from build123d import *

# Parameters (mm, degrees)
F0_W     = 139.677039
F0_H     = 166.199392
F1_DEPTH = 13
F3_DEPTH = 8


# Not quite as in the source:
# - ends of sketch curves that miss each other by under 0.0002 mm in the source are joined


with BuildPart() as f1:
    # F0 (on Top) → F1 (new body)
    with BuildSketch(Plane.XY):
        with Locations((5e-07, 0)):
            Rectangle(F0_W, F0_H)
    extrude(amount=F1_DEPTH)

    # F2 (on face) → F3 (cut)
    with BuildSketch(Plane.XY.offset(13)):
        with BuildLine():
            Line((-52.224, 63.413361), (-52.224, -19.296639))
            ThreePointArc((-52.224, -19.296639), (-23.4870244983, -65.9411012245), (31.0980686358, -61.2520475086))
            Line((31.0980686358, -61.2520475086), (46.412829, -75.243303))
            Line((46.412829, -75.243303), (60.220039, -60.767602))
            Line((60.220039, -60.767602), (44.587774, -46.486281))
            ThreePointArc((44.587774, -46.486281), (50.2787135157, -33.4174443314), (52.224, -19.296639))
            Line((52.224, -19.296639), (52.224, 63.413361))
            Line((52.224, 63.413361), (35, 63.413361))
            Line((35, 63.413361), (35, -19.296639))
            ThreePointArc((35, -19.296639), (34.1157796878, -27.1141562719), (31.5077956402, -34.536678826))
            Line((31.5077956402, -34.536678826), (17.818477, -22.030395))
            Line((17.818477, -22.030395), (4.000974, -36.496692))
            Line((4.000974, -36.496692), (18.018091, -49.302445))
            ThreePointArc((18.018091, -49.302445), (-17.2390082984, -49.756720958), (-35, -19.296639))
            Line((-35, -19.296639), (-35, 63.413361))
            Line((-35, 63.413361), (-52.224, 63.413361))
        make_face()
    extrude(amount=-F3_DEPTH, mode=Mode.SUBTRACT)


solid = f1.part
Design review of the part built by this model. Coordinates are the model's own, in mm. A direction names the side the tool comes from. Coordinates: 2 decimals unless noted, no trailing zeros. Write each loop counter-clockwise with the first axis right and the second up, starting at its lowest first coordinate (ties: lowest second). Pieces come first, ordered by that corner, then holes. Notation, with made-up numbers: (18, 22) - (59, 22) arc R21 ccw to (59, 57) - close; hole circle Ø9 at (72, -7). An arc over 180 degrees is marked (long way). One line per item, written item: value.
1) Add section A-A (z = 11.25). State the section outline as (x, y) points, plus the area to 3 significant figures.
Answer sheet:
outline: (-69.84, -83.1) - (69.84, -83.1) - (69.84, 83.1) - (-69.84, 83.1) - close; hole (-52.22, -19.3) arc R52.22 ccw to (31.1, -61.25) - (46.41, -75.24) - (60.22, -60.77) - (44.59, -46.49) arc R52.22 ccw to (52.22, -19.3) - (52.22, 63.41) - (35, 63.41) - (35, -19.3) arc R35 cw to (31.51, -34.54) - (17.82, -22.03) - (4, -36.5) - (18.02, -49.3) arc R35 cw to (-35, -19.3) - (-35, 63.41) - (-52.22, 63.41) - close
area: 17,200 mm2
2) Insertion check: pin 1 (4 mm diameter, centred on x = -38.5, y = 57.5, fed in from +Z). The pin has a flat end and moves straight along its axis. Give the tip position at first contact, or say it passes through.
Answer sheet:
pin 1: stops at z = 5
3) Mouldability with a two-part tool opening along Y and no side actions: class faces 3 (the face through (-1, 1, 0)), 4 (the face through (-1, -83.1, 6)), 5 (the face through (44, 63.413, 9)) as +Y half, -Y half, draft (parallel to the pull), parting line (faces both ways), or undercut.
Answer sheet:
face 3: draft
face 4: -Y half
face 5: undercut
4) For faces 1 (the face through (-69.839, -1, 6)), 2 (the face through (-43, 63.413, 9)), list the 3-axis set-ups (+Z, -Z, +X, -X, +Y, -Y) from which the entire face can be reached by the end or side of a thin tool; tool diameter is ignored.
Answer sheet:
face 1: +Z, -Z, -X, +Y, -Y
face 2: +Z
5) Add section C-C (x = 38.5). State the section outline as (y, z) points.
Answer sheet:
outline: (-83.1, 0) - (83.1, 0) - (83.1, 13) - (63.41, 13) - (63.41, 5) - (-68.01, 5) - (-68.01, 13) - (-83.1, 13) - close
6) Add section B-B (y = 3.5). State the section outline as (x, z) points.
Answer sheet:
outline: (-69.84, 0) - (69.84, 0) - (69.84, 13) - (52.22, 13) - (52.22, 5) - (35, 5) - (35, 13) - (-35, 13) - (-35, 5) - (-52.22, 5) - (-52.22, 13) - (-69.84, 13) - close
7) To check wall thickness, follow probe 1 along Y at (x, z) = (-0.5, 7.75); probe 2 along X at (y, z) = (-32, 8.75); probe 3 along Z at (x, y) = (-2.5, -61.5). State the ranges of each line that lie inside material, in increasing order.
Answer sheet:
probe 1: y = -83.1 to -71.52, -54.29 to 83.1
probe 2: x = -69.84 to -50.66, -32.61 to 8.3, 28.73 to 32.61, 50.66 to 69.84
probe 3: z = 0 to 5
8) Add section D-D (x = -45.5). State the section outline as (y, z) points, plus the area to 3 significant figures.
Answer sheet:
outline: (-83.1, 0) - (83.1, 0) - (83.1, 13) - (63.41, 13) - (63.41, 5) - (-44.93, 5) - (-44.93, 13) - (-83.1, 13) - close
area: 1,290 mm2
